Can you work these out from the model? Positions are in its coordinate system, mm. Face numbers are marked on the shaded views. A direction names the side the tool comes from. Coordinates: 2 decimals unless noted, no trailing zeros. Write each loop counter-clockwise with the first axis right and the second up, starting at its lowest first coordinate (ties: lowest second). Pieces come first, ordered by that corner, then holes.
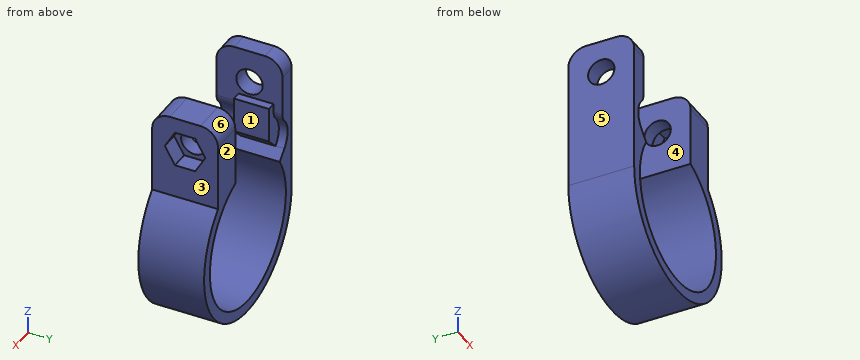
```python
from build123d import *

# Parameters (mm, degrees)
PAD_DEPTH       = 15
SKETCH001_R     = 3
POCKET_DEPTH    = 38.001
FILLET_R        = 4
POCKET001_DEPTH = 4
POCKET002_DEPTH = 5
POCKET003_DEPTH = 2


with BuildPart() as part:
    # Sketch → Pad (new body)
    with BuildSketch(Plane.XZ):
        with BuildLine():
            Line((-19, 0), (-19, 33))
            Line((-19, 33), (-15, 33))
            Line((-15, 33), (-15, 21.856406))
            Line((-15, 21.856406), (-13, 21.856406))
            Line((-13, 21.856406), (-13, 13.856406))
            Line((-13, 13.856406), (-15.828427, 11.027979))
            Line((-15.828427, 11.027979), (-13.817926, 9.017478))
            ThreePointArc((-13.817926, 9.017478), (5.303714, -15.62436), (5.473078, 15.565841))
            Line((5.473078, 15.565841), (5.473078, 33))
            Line((5.473078, 33), (12.973078, 33))
            Line((12.973078, 33), (12.973078, 13.881615))
            ThreePointArc((-19, 0), (7.566753, -17.42826), (12.973078, 13.881615))
        make_face()
    extrude(amount=PAD_DEPTH)

    # Sketch001 (on Face1 of Pad) → Pocket (cut, through all)
    with BuildSketch(Plane(origin=(-19, 0, 0), x_dir=(0, 0, -1), z_dir=(-1, 0, 0))):
        with Locations((-25.5, 7.5)):
            Circle(SKETCH001_R)
    extrude(amount=-POCKET_DEPTH, mode=Mode.SUBTRACT)

    # Fillet
    fillet_edges = [part.edges().sort_by_distance(p)[0] for p in [
        (-17, 0, 33),
        (-17, -15, 33),
        (9.223078, -15, 33),
        (9.223078, 0, 33),
    ]]
    fillet(fillet_edges, radius=FILLET_R)

    # Sketch002 (on Face10 of Fillet) → Pocket001 (cut)
    with BuildSketch(Plane(origin=(12.973078, 0, 0), x_dir=(0, 0, 1), z_dir=(1, 0, 0))):
        Polygon((21.5, 9.809401), (21.5, 5.190599), (25.5, 2.881198), (29.5, 5.190599), (29.5, 9.809401), (25.5, 12.118802), align=None)
    extrude(amount=-POCKET001_DEPTH, mode=Mode.SUBTRACT)

    # Sketch003 (on Face6 of Pocket001) → Pocket002 (cut)
    with BuildSketch(Plane.XZ.offset(15)):
        with BuildLine():
            Line((-15, 21.856406), (-15, 19.856406))
            ThreePointArc((-15.828427, 17.856406), (-15.215301, 18.774014), (-15, 19.856406))
            ThreePointArc((-15.828427, 17.856406), (-17.242641, 14.442193), (-15.828427, 11.027979))
            Line((-13, 13.856406), (-15.828427, 11.027979))
            Line((-13, 21.856406), (-13, 13.856406))
            Line((-15, 21.856406), (-13, 21.856406))
        make_face()
    extrude(amount=-POCKET002_DEPTH, mode=Mode.SUBTRACT)

    # Sketch004 (on Face2 of Pocket002) → Pocket003 (cut)
    with BuildSketch(Plane(origin=(0, 0, 0), x_dir=(1, 0, 0), z_dir=(0, 1, 0))):
        with BuildLine():
            Line((-15, -21.856406), (-15, -19.856406))
            ThreePointArc((-15, -19.856406), (-15.215301, -18.774014), (-15.828427, -17.856406))
            ThreePointArc((-15.828427, -11.027979), (-17.242641, -14.442193), (-15.828427, -17.856406))
            Line((-13, -13.856406), (-15.828427, -11.027979))
            Line((-13, -21.856406), (-13, -13.856406))
            Line((-15, -21.856406), (-13, -21.856406))
        make_face()
    extrude(amount=-POCKET003_DEPTH, mode=Mode.SUBTRACT)


solid = part.part
```
1. We'd pull the mould along X, two halves only. Please class the marked faces 4, 5 and 6: released by +X, released by -X, zero draft, split by the parting line, or undercut.
2. If we section it at A-A, the plane y = -7.5: List the corners of the cut face in (x, z) for me, plus the area to 3 significant figures.
3. If we section it at B-B, the plane z = -6: List the corners of the cut face in (x, y) for me.
4. If we section it at D-D, the plane z = 14.5: List the corners of the cut face in (x, y) for me.
5. If we section it at C-C, the plane x = 0: List the corners of the cut face in (y, z) for me.
6. If I drill on L1, parallel to X at y = -6.25, z = 18; L2, parallel to Y at x = 8.1, z = 25.5; L3, parallel to Z at x = 8.1, y = -7.5, over which ranges is the centre line in solid material (lowest first)?
7. I'm going to push flat-ended pins straight in: P1, Ø6.5, axis at y = -10.5, z = 26, coming from the +X side; P2, Ø2, axis at x = -15.5, z = 16.5, coming from the -Y side; P3, Ø1.5, axis at x = -5, y = -11, coming from the -Z side. Where does each tip first touch, or does it pass through?
8. Which directions (+Z, -Z, +X, -X, +Y, -Y) give clear straight access to the entire face, cutting with the end or side of a thin tool? Please do the marked faces 1, 2 and 3.
Answers:
1. face 4: undercut
1. face 5: released by -X
1. face 6: zero draft
2. outline: (-19, 0) arc R19 ccw (long way) to (12.97, 13.88) - (12.97, 21.5) - (8.97, 21.5) - (8.97, 22.5) - (5.47, 22.5) - (5.47, 15.57) arc R16.5 cw (long way) to (-13.82, 9.02) - (-15.83, 11.03) - (-13, 13.86) - (-13, 21.86) - (-15, 21.86) - (-15, 22.5) - (-19, 22.5) - close; (-19, 28.5) - (-15, 28.5) - (-15, 33) - (-19, 33) - close; (5.47, 28.5) - (8.97, 28.5) - (8.97, 29.5) - (12.97, 29.5) - (12.97, 33) - (5.47, 33) - close
2. area: 387 mm2
3. outline: (-18.03, -15) - (-15.37, -15) - (-15.37, 0) - (-18.03, 0) - close; (15.37, -15) - (18.03, -15) - (18.03, 0) - (15.37, 0) - close
4. outline: (-19, -15) - (-17.24, -15) - (-17.24, -10) - (-13, -10) - (-13, -2) - (-17.24, -2) - (-17.24, 0) - (-19, 0) - close; (7.87, -15) - (12.97, -15) - (12.97, 0) - (7.87, 0) - close
5. outline: (-15, -19) - (0, -19) - (0, -16.5) - (-15, -16.5) - close
6. L1: x = -19 to -13, 5.47 to 12.97
6. L2: y = -15 to -10.5, -4.5 to 0
6. L3: z = -17.19 to -14.37, 14.37 to 22.5, 28.5 to 33
7. P1: stops at x = 12.97
7. P2: stops at y = -10
7. P3: stops at z = -18.52
8. face 1: +Z, +Y, -Y
8. face 2: +Z, -Z, +X, -X, +Y
8. face 3: +Z, +X, +Y, -Y
